Design review of the part built by this model. Coordinates are the model's own, in mm. A direction names the side the tool comes from. Coordinates: 2 decimals unless noted, no trailing zeros. Write each loop counter-clockwise with the first axis right and the second up, starting at its lowest first coordinate (ties: lowest second). Pieces come first, ordered by that corner, then holes. Notation, with made-up numbers: M 86.5,30.5 L 122.5,30.5 A27 ccw 122.5,52.5 Z; hole C 20,14 d4. An arc over 180 degrees is marked long. Write each question's results on one line, items separated by ' | '. Start each with the question number.
```python
from build123d import *

# Parameters (mm, degrees)
SKETCH1_W                 = 30
SKETCH1_H                 = 30
SKETCH1_R                 = 14
BOSS_EXTRUDE1_DEPTH       = 8
SKETCH2_R                 = 5
BOSS_EXTRUDE2_DEPTH       = 8
BOSS_EXTRUDE3_DEPTH       = 2
F_2_0MM_DOWEL_HOLE1_D     = 2
F_2_0MM_DOWEL_HOLE1_DEPTH = 8
SKETCH7_R                 = 6
BOSS_EXTRUDE4_DEPTH       = 5
BOSS_EXTRUDE5_DEPTH       = 12
CIRPATTERN1_COUNT         = 7


with BuildPart() as part:
    # Sketch1 → Boss-Extrude1 (new body)
    with BuildSketch(Plane(origin=(0, 0, 0), x_dir=(1, 0, 0), z_dir=(0, 1, 0))):
        Rectangle(SKETCH1_W, SKETCH1_H)
        Circle(SKETCH1_R, mode=Mode.SUBTRACT)
    extrude(amount=BOSS_EXTRUDE1_DEPTH)



with BuildPart() as body_2:
    # Sketch2 → Boss-Extrude2 (new body)
    with BuildSketch(Plane(origin=(0, 0, 0), x_dir=(1, 0, 0), z_dir=(0, 1, 0))):
        Circle(SKETCH2_R)
    extrude(amount=BOSS_EXTRUDE2_DEPTH)


with BuildPart() as part_1:
    add(part.part)

    add(body_2.part)  # Boss-Extrude3 merges body 2
    # Sketch3 → Boss-Extrude3 (add)
    with BuildSketch(Plane(origin=(0, 8, 0), x_dir=(1, 0, 0), z_dir=(0, 1, 0))):
        with BuildLine():
            Line((-1, 5), (-1, 14))
            ThreePointArc((-1, 14), (0, 15), (1, 14))
            Line((1, 14), (1, 5))
            ThreePointArc((1, 5), (0, 4), (-1, 5))
        make_face()
        with BuildLine():
            Line((-3.830127019, -3.366025404), (-11.624355653, -7.866025404))
            ThreePointArc((-11.624355653, -7.866025404), (-12.990381057, -7.5), (-12.624355653, -6.133974596))
            Line((-12.624355653, -6.133974596), (-4.830127019, -1.633974596))
            ThreePointArc((-4.830127019, -1.633974596), (-3.464101615, -2), (-3.830127019, -3.366025404))
        make_face()
        with BuildLine():
            Line((4.830127019, -1.633974596), (12.624355653, -6.133974596))
            ThreePointArc((12.624355653, -6.133974596), (12.990381057, -7.5), (11.624355653, -7.866025404))
            Line((11.624355653, -7.866025404), (3.830127019, -3.366025404))
            ThreePointArc((3.830127019, -3.366025404), (3.464101615, -2), (4.830127019, -1.633974596))
        make_face()
    extrude(amount=-BOSS_EXTRUDE3_DEPTH)

    # Ø2.0mm Dowel Hole1
    with Locations(Plane(origin=(0, 8, 0), x_dir=(1, 0, 0), z_dir=(0, 1, 0))):
        with Locations((13, 13), (-13, 13), (-13, -13), (13, -13)):
            Hole(F_2_0MM_DOWEL_HOLE1_D / 2, depth=F_2_0MM_DOWEL_HOLE1_DEPTH)

    # Sketch7 → Boss-Extrude4 (add)
    with BuildSketch(Plane.XZ):
        Circle(SKETCH7_R)
    extrude(amount=-BOSS_EXTRUDE4_DEPTH)

    # Sketch9 → Boss-Extrude5 (add)
    with BuildSketch(Plane.XY):
        Polygon((0, 5), (-4.898979486, 0), (-4.498979486, 0), (0.4, 5), align=None)
    boss_extrude5 = extrude(amount=BOSS_EXTRUDE5_DEPTH)

    # CirPattern1: Boss-Extrude5 ×7 about axis
    cirpattern1_axis = Axis((0, 0, 0), (0, 1, 0))
    for i in range(1, CIRPATTERN1_COUNT):
        add(boss_extrude5.rotate(cirpattern1_axis, i * 360 / CIRPATTERN1_COUNT))


solid = part_1.part
```
Item 1: Insertion check: pin 1 Ø1.6 at (x, z) = (-13, -13) entering from +Y. The pin has a flat end and moves straight along its axis. Give the tip position at first contact, or say it passes through.
Item 2: For faces 1 (the cylindrical face through (2.307, 6.479, 4.436)), 2 (the flat face through (7.77, 7.01, 5.64)), list the 3-axis set-ups (+Z, -Z, +X, -X, +Y, -Y) from which the entire face can be reached by the end or side of a thin tool; tool diameter is ignored.
Item 3: We need section D-D on z = 13. State the section outline as (x, y) points, then the cut area to 3 significant figures.
Item 4: We need section C-C on y = 7.25. State the section outline as (x, z) points.
Item 5: We need section A-A on y = 5.5. State the section outline as (x, z) points, then the cut area to 3 significant figures.
Item 6: Wall thickness on L1, parallel to Z at x = 0, y = 5.25; L2, parallel to X at y = 2.75, z = 4.25; L3, parallel to X at y = 4.25, z = 10: over which ranges is each line inside the solid? List them lowest first.
Item 7: We need section B-B on x = 8.75. State the section outline as (y, z) points, then the cut area to 3 significant figures.
Item 8: Draft analysis for pull direction X (two halves, no side actions). For faces 3 (the cylindrical face through (13, 4, -12)), 4 (the flat face through (-15, 4, 0)), state which applies: released by +X, released by -X, zero draft, split by the parting line, or undercut.
Answer:
1) pin 1: passes through
2) face 1: none | face 2: +Y
3) outline: M -15,0 L -14,0 L -14,8 L -15,8 Z; M -12,0 L -5.2,0 L -5.2,8 L -12,8 Z; M 5.2,0 L 12,0 L 12,8 L 5.2,8 Z; M 14,0 L 15,0 L 15,8 L 14,8 Z | area: 125 mm^2
4) outline: M -15,-15 L 15,-15 L 15,15 L -15,15 Z; hole C -13,-13 d2; hole C -13,13 d2; hole M -12.59,6.12 A14 ccw -1,-13.96 L -1,-5 A1 cw -0.99,-4.9 A5 cw -4.74,1.59 A1 cw -4.83,1.63 Z; hole M -11.59,7.85 L -3.83,3.37 A1 cw -3.75,3.31 A5 cw 3.75,3.31 A1 cw 3.83,3.37 L 11.59,7.85 A14 ccw Z; hole M 0.99,-4.9 A1 cw 1,-5 L 1,-13.96 A14 ccw 12.59,6.12 L 4.83,1.63 A1 cw 4.74,1.59 A5 cw Z; hole C 13,-13 d2; hole C 13,13 d2
5) outline: M -15,-15 L 15,-15 L 15,15 L -15,15 Z; C 0,0 d10; hole C -13,-13 d2; hole C 0,0 d28; hole C -13,13 d2; hole C 13,-13 d2; hole C 13,13 d2 | area: 350 mm^2
6) L1: z = -15 to -14, -5 to 5, 14 to 15 | L2: x = -15 to -13.34, -8.87 to -8.22, -4.24 to 4.24, 13.34 to 15 | L3: x = -15 to -9.8, -0.73 to -0.33, 9.8 to 15
7) outline: M 0,-15 L 8,-15 L 8,-10.93 L 0,-10.93 Z; M 0,-7.8 L 0.58,-9.11 L 0.99,-9.11 L 0,-6.88 Z; M 0,2.62 L 5,-2.41 L 5,-2 L 0,3.03 Z; M 0,10.93 L 8,10.93 L 8,15 L 0,15 Z; M 3.56,8.27 L 5,6.47 L 5,6.98 L 3.97,8.27 Z; M 6,3.9 L 8,3.9 L 8,6.21 L 6,6.21 Z | area: 73.2 mm^2
8) face 3: undercut | face 4: released by -X
